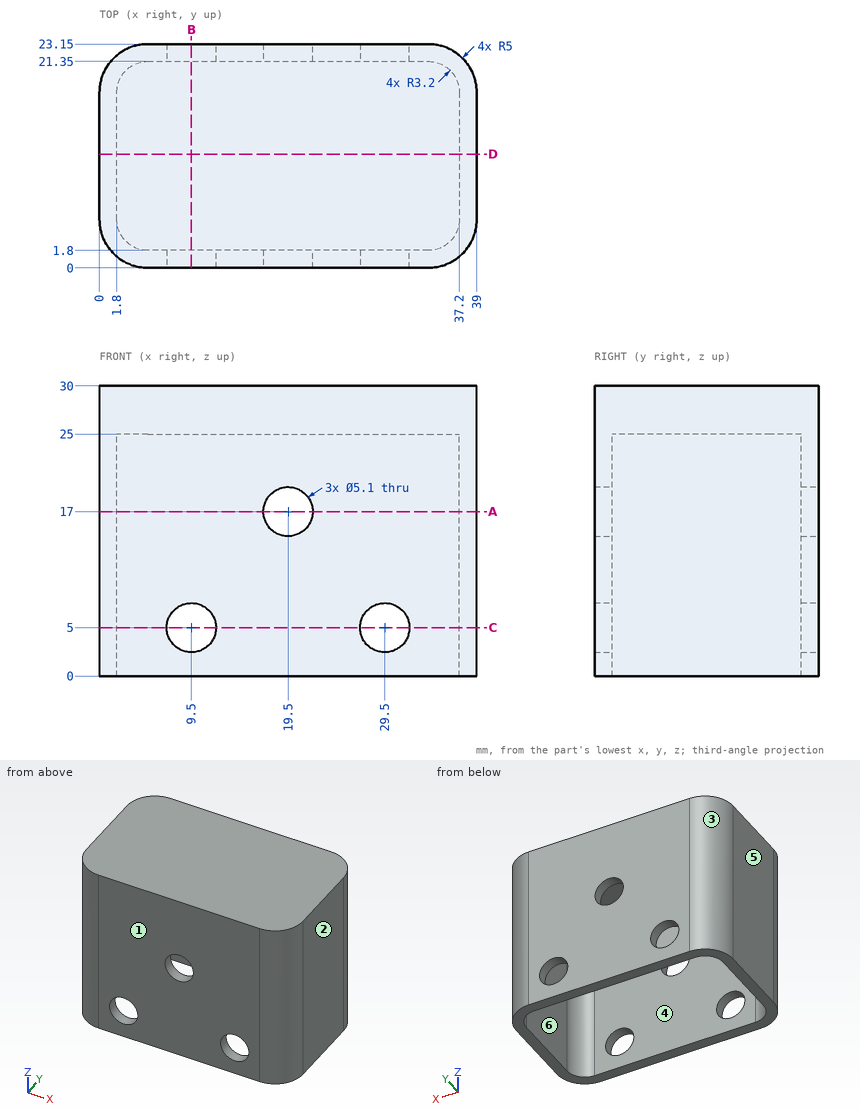
Answer from the drawing. Dimensions are ordinates in mm from the lowest x, y and z of the part. A direction names the side the tool comes from. Coordinates: 2 decimals unless noted, no trailing zeros. Loops run counter-clockwise (first coordinate to the right, second up) from the corner with the lowest first, then second, coordinate; pieces in that order, holes last.
Q1. Each of these flat-tipped pins is pushed along its axis until it touches: pin 1 Ø4 at (x, z) = (19.5, 17) entering from -Y; pin 2 Ø8 at (x, z) = (29.5, 5) entering from +Y; pin 3 Ø1.5 at (x, y) = (23, 9) entering from -Z. Where does it stop, or does it pass through?
Q2. The part is cut by section D-D on y = 11.75. Write down the section's boundary in (x, z), and give its area (3 significant figures).
Q3. The part is cut by section C-C on z = 5. Give the number of separate pieces and of enclosed holes in the cut face, and give its area (3 significant figures).
Q4. The part is cut by section B-B on x = 9.5. Write down the section's boundary in (y, z), and give its area (3 significant figures).
Q5. Which of the six approach directions +Z, -Z, +X, -X, +Y, -Y give full straight-line access (tool end or side, diameter ignored) to the marked faces 5 and 6?
Q6. The mould has two halves that part along Y. Classify the marked faces 1, 2, 3 and 4: +Y half, -Y half, draft (parallel to the pull), parting line (faces both ways), or undercut.
Q7. Consider probe 1 along Y at (x, z) = (30.5, 18.75); probe 2 along Z at (x, y) = (29.5, 1.1); probe 3 along X at (y, z) = (6.25, 11.5). Determine where each line is inside the solid, lowest interval first.
Q8. The part is cut by section A-A on z = 17. Write down the section's boundary in (x, y), and give its area (3 significant figures).
Results below:
1. pin 1: passes through
1. pin 2: stops at y = 23.15
1. pin 3: stops at z = 25
2. outline: (0, 0) - (1.8, 0) - (1.8, 25) - (37.2, 25) - (37.2, 0) - (39, 0) - (39, 30) - (0, 30) - close
2. area: 285 mm2
3. separate pieces: 4
3. enclosed holes: 0
3. area: 161 mm2
4. outline: (0, 0) - (1.8, 0) - (1.8, 2.45) - (0, 2.45) - close; (0, 7.55) - (1.8, 7.55) - (1.8, 25) - (21.35, 25) - (21.35, 7.55) - (23.15, 7.55) - (23.15, 30) - (0, 30) - close; (21.35, 0) - (23.15, 0) - (23.15, 2.45) - (21.35, 2.45) - close
4. area: 187 mm2
5. face 5: +Z, -Z, -X, +Y, -Y
5. face 6: -Z
6. face 1: -Y half
6. face 2: draft
6. face 3: +Y half
6. face 4: undercut
7. probe 1: y = 0 to 1.8, 21.35 to 23.15
7. probe 2: z = 0 to 2.45, 7.55 to 30
7. probe 3: x = 0 to 1.8, 37.2 to 39
8. outline: (0, 5) arc R5 ccw to (5, 0) - (16.95, 0) - (16.95, 1.8) - (5, 1.8) arc R3.2 cw to (1.8, 5) - (1.8, 18.15) arc R3.2 cw to (5, 21.35) - (16.95, 21.35) - (16.95, 23.15) - (5, 23.15) arc R5 ccw to (0, 18.15) - close; (22.05, 0) - (34, 0) arc R5 ccw to (39, 5) - (39, 18.15) arc R5 ccw to (34, 23.15) - (22.05, 23.15) - (22.05, 21.35) - (34, 21.35) arc R3.2 cw to (37.2, 18.15) - (37.2, 5) arc R3.2 cw to (34, 1.8) - (22.05, 1.8) - close
8. area: 180 mm2
